```python
from build123d import *

# Parameters (mm, degrees)
SKETCH_1_W             = 250
SKETCH_1_H             = 250
SM_BASE_FLANGE_1_DEPTH = 8
CUT_EXTRUDE_1_DEPTH    = 10
CUT_EXTRUDE_2_DEPTH    = 10


# Sheet-metal steps are written as plain solids
with BuildPart() as part:
    # Sketch 1 → Базовая кромка1 (new body)
    with BuildSketch(Plane.XY):
        with Locations((125, -125)):
            Rectangle(SKETCH_1_W, SKETCH_1_H)
    extrude(amount=-SM_BASE_FLANGE_1_DEPTH)

    # Sketch 2 → Вырез-Вытянуть1 (cut)
    with BuildSketch(Plane.XY):
        Polygon((52.778688881, 0), (0, -72.9), (0, 0), align=None)
        Polygon((250, 0), (197.221311119, 0), (250, -72.9), align=None)
        Polygon((197.221311119, -250), (250, -177.1), (250, -250), align=None)
        Polygon((0, -250), (52.778688881, -250), (0, -177.1), align=None)
    extrude(amount=-CUT_EXTRUDE_1_DEPTH, mode=Mode.SUBTRACT)

    # Эскиз3 → Вырез-Вытянуть2 (cut)
    with BuildSketch(Plane(origin=(0, 0, -8), x_dir=(-1, 0, 0), z_dir=(0, 0, -1))):
        with BuildLine():
            Line((-65.757289426, -29.819990865), (-56.960841279, -41.969990865))
            ThreePointArc((-56.960841279, -41.969990865), (-58.525832144, -51.745), (-68.300841279, -50.180009135))
            Line((-68.300841279, -50.180009135), (-77.097289426, -38.030009135))
            ThreePointArc((-77.097289426, -38.030009135), (-75.532298561, -28.255), (-65.757289426, -29.819990865))
        make_face()
        with BuildLine():
            Line((-42.300094368, -62.219990865), (-33.503646221, -74.369990865))
            ThreePointArc((-33.503646221, -74.369990865), (-35.068637085, -84.145), (-44.843646221, -82.580009135))
            Line((-44.843646221, -82.580009135), (-53.640094368, -70.430009135))
            ThreePointArc((-53.640094368, -70.430009135), (-52.075103503, -60.655), (-42.300094368, -62.219990865))
        make_face()
        with BuildLine():
            Line((-184.242710574, -29.819990865), (-193.039158721, -41.969990865))
            ThreePointArc((-193.039158721, -41.969990865), (-191.474167856, -51.745), (-181.699158721, -50.180009135))
            Line((-181.699158721, -50.180009135), (-172.902710574, -38.030009135))
            ThreePointArc((-172.902710574, -38.030009135), (-174.467701439, -28.255), (-184.242710574, -29.819990865))
        make_face()
        with BuildLine():
            Line((-207.699905632, -62.219990865), (-216.496353779, -74.369990865))
            ThreePointArc((-216.496353779, -74.369990865), (-214.931362915, -84.145), (-205.156353779, -82.580009135))
            Line((-205.156353779, -82.580009135), (-196.359905632, -70.430009135))
            ThreePointArc((-196.359905632, -70.430009135), (-197.924896497, -60.655), (-207.699905632, -62.219990865))
        make_face()
        with BuildLine():
            Line((-65.757289426, -220.180009135), (-56.960841279, -208.030009135))
            ThreePointArc((-56.960841279, -208.030009135), (-58.525832144, -198.255), (-68.300841279, -199.819990865))
            Line((-68.300841279, -199.819990865), (-77.097289426, -211.969990865))
            ThreePointArc((-77.097289426, -211.969990865), (-75.532298561, -221.745), (-65.757289426, -220.180009135))
        make_face()
        with BuildLine():
            Line((-42.300094368, -187.780009135), (-33.503646221, -175.630009135))
            ThreePointArc((-33.503646221, -175.630009135), (-35.068637085, -165.855), (-44.843646221, -167.419990865))
            Line((-44.843646221, -167.419990865), (-53.640094368, -179.569990865))
            ThreePointArc((-53.640094368, -179.569990865), (-52.075103503, -189.345), (-42.300094368, -187.780009135))
        make_face()
        with BuildLine():
            Line((-184.242710574, -220.180009135), (-193.039158721, -208.030009135))
            ThreePointArc((-193.039158721, -208.030009135), (-191.474167856, -198.255), (-181.699158721, -199.819990865))
            Line((-181.699158721, -199.819990865), (-172.902710574, -211.969990865))
            ThreePointArc((-172.902710574, -211.969990865), (-174.467701439, -221.745), (-184.242710574, -220.180009135))
        make_face()
        with BuildLine():
            Line((-207.699905632, -187.780009135), (-216.496353779, -175.630009135))
            ThreePointArc((-216.496353779, -175.630009135), (-214.931362915, -165.855), (-205.156353779, -167.419990865))
            Line((-205.156353779, -167.419990865), (-196.359905632, -179.569990865))
            ThreePointArc((-196.359905632, -179.569990865), (-197.924896497, -189.345), (-207.699905632, -187.780009135))
        make_face()
    extrude(amount=-CUT_EXTRUDE_2_DEPTH, mode=Mode.SUBTRACT)


solid = part.part
```
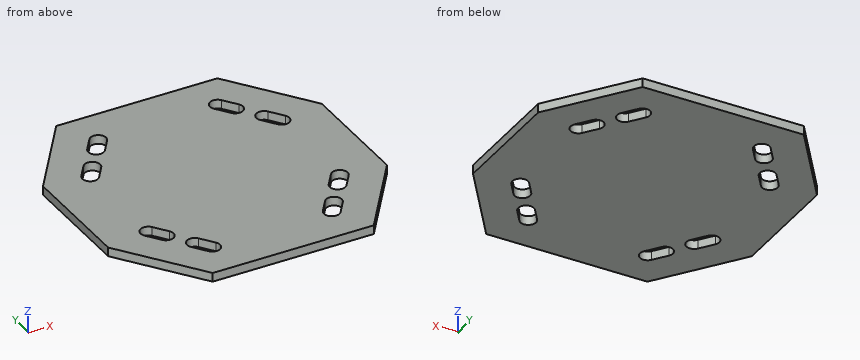
Geometry check sheet. Reference: the model listing, model coordinates, mm. Coordinates: 2 decimals unless noted, no trailing zeros. Write each loop counter-clockwise with the first axis right and the second up, starting at its lowest first coordinate (ties: lowest second). Pieces come first, ordered by that corner, then holes. Notation, with made-up numbers: M -28,32.5 L -16,32.5 A21 cw -16,67.5 Z; hole C 61,57.5 d3. An arc over 180 degrees is marked long. Use one line per item in the form item = value. Start each with the question number.
1) Section check D-D on x = 226. Enter the section's corners in (y, z).
2) Section check B-B on x = 38. Enter the section's corners in (y, z).
3) Section check A-A on y = -33.5. Enter the section's corners in (x, z), and give its area (3 significant figures).
4) Section check C-C on z = -4.25. State how many separate pieces and enclosed holes the cut face has, and give its area (3 significant figures).
5) Thickness scan on probe 1 along X at (y, z) = (-47, -1); probe 2 along X at (y, z) = (-218, -3); probe 3 along Y at (x, z) = (37, -7.5). Record the ranges inside material, lowest first. Write a range as from..to.
Responses:
q1.outline = M -210.25,-8 L -39.75,-8 L -39.75,0 L -210.25,0 Z
q2.outline = M -229.59,-8 L -181.84,-8 L -181.84,0 L -229.59,0 Z; M -164.62,-8 L -85.38,-8 L -85.38,0 L -164.62,0 Z; M -68.16,-8 L -20.41,-8 L -20.41,0 L -68.16,0 Z
q3.outline = M 28.53,-8 L 63.09,-8 L 63.09,0 L 28.53,0 Z; M 78.41,-8 L 171.59,-8 L 171.59,0 L 78.41,0 Z; M 186.91,-8 L 221.47,-8 L 221.47,0 L 186.91,0 Z
q3.area = 1,300 mm2
q4.separate_pieces = 1
q4.enclosed_holes = 8
q4.area = 51,900 mm2
q5.probe_1 = 18.75..55.69, 70.6..179.4, 194.31..231.25
q5.probe_2 = 29.61..64.18, 78.16..171.84, 185.82..220.39
q5.probe_3 = -228.21..-180.46, -164.87..-85.13, -69.54..-21.79
